from build123d import *

# Parameters (mm, degrees)
F0_R     = 1.075
F1_DEPTH = 50
F3_DEPTH = 50


with BuildPart() as f1:
    # F0 (on Front) → F1 (new body)
    with BuildSketch(Plane.XZ):
        Polygon((25, -25), (50, -25), (50, 25), (-50, 25), (-80, -25), (-50, -25), align=None)
        with Locations((-50, -17)):
            Circle(F0_R, mode=Mode.SUBTRACT)
        with Locations((25.408758, -17)):
            Circle(F0_R, mode=Mode.SUBTRACT)
    extrude(amount=F1_DEPTH)

    # F2 (on face) → F3 (cut)
    with BuildSketch(Plane.XZ.offset(50)):
        Polygon((-50, 25), (-65, 0), (-28.095694, -4.829377), (-5.397624, 7.244065), (15.610165, 7.244065), (50, 16.178414), (50, 25), align=None)
    extrude(amount=-F3_DEPTH, mode=Mode.SUBTRACT)


solid = f1.part
Geometry: final body of the model. Coordinates: model frame, mm. A direction names the side the tool comes from. Give positions to 0.01 mm unless a question says otherwise; leave off trailing zeros. Loops run counter-clockwise (first coordinate to the right, second up) from the corner with the lowest first, then second, coordinate; pieces in that order, holes last. Notation, with made-up numbers: M 87.25,62 L 141.25,62 A18 ccw 141.25,97 Z; hole C 54.25,22.25 d11. An arc over 180 degrees is marked long. Put each result on its own line as item: value. Start each with the question number.
1) Contact query for flat-ended pins moving along their axis: pin 1 (6.5 mm diameter, centred on x = 4.5, y = -37, fed in from +Z); pin 2 (1.9 mm diameter, centred on x = -50, z = -17, fed in from +Y); pin 3 (6 mm diameter, centred on x = 26, y = -39, fed in from +Z); pin 4 (2 mm diameter, centred on x = -40.5, y = -36.5, fed in from +Z). Output: stop coordinate, or through.
2) Ray query, line 1 along Z through (x, y) = (4.5, -12); line 2 along Z through (x, y) = (-50, -25) (3 decimals); line 3 along Z through (x, y) = (-26.5, -16.5). Return the intervals inside material, ascending.
3) Cut plane B-B (z = -14). Output: boundary loops of the cut face in (x, y).
4) Cut plane A-A (y = -32). Output: boundary loops of the cut face in (x, z) (3 decimals).
5) Access query for faces 4 (the flat face through (5, -25, 7.244)), 5 (the flat face through (-46.81, -25.35, -2.38)), 6 (the flat face through (-16, -25, -25)). Directions: +Z, -Z, +X, -X, +Y, -Y. A direction counts if a zero-diameter tool reaches every point of the face in a straight line with its end or side. Return the directions, or none.
6) Pull-direction query (X, two-part tool) for faces 1 (the flat face through (-16.91, -25.35, 1.12)), 2 (the flat face through (-1, -50, -9)), 3 (the flat face through (32.564, -25.35, 11.649)); classes: pulls with the +X half, pulls with the -X half, needs draft (parallel to the pull), parting line crosses it, or undercut.
7) Cut plane C-C (x = 6.5). Output: boundary loops of the cut face in (y, z), then the cut area to 3 significant figures.
Verdict:
1. pin 1: z = 7.24
1. pin 2: through
1. pin 3: z = 10.72
1. pin 4: z = -3.08
2. line 1: -25 to 7.24
2. line 2: -25 to -18.075, -15.925 to -1.963
2. line 3: -25 to -3.98
3. outline: M -73.4,-50 L 50,-50 L 50,0 L -73.4,0 Z
4. outline: M -80,-25 L 50,-25 L 50,16.178 L 15.61,7.244 L -5.398,7.244 L -28.096,-4.829 L -65,0 Z; hole C -50,-17 d2.15; hole C 25.409,-17 d2.15
5. face 4: +Z, -X, +Y, -Y
5. face 5: +Z, +Y, -Y
5. face 6: -Z, +X, -X, +Y, -Y
6. face 1: undercut
6. face 2: needs draft
6. face 3: pulls with the -X half
7. outline: M -50,-25 L 0,-25 L 0,7.24 L -50,7.24 Z
7. area: 1,610 mm2
